Could you check a few things on this model? Use its own coordinates, in mm. Round coordinates to 2 decimals unless told otherwise and drop trailing zeros. Order: outer loops, then holes, each group sorted by start corner. A loop starts at its lowest first (then second) coordinate and runs counter-clockwise, first axis right, second up. Notation, with made-up numbers: (-23.75, -40) -> (-11.75, -40) arc R9 cw to (-11.75, -25) -> close; hole circle Ø6 at (-1, -37.75). An arc over 180 degrees is marked (long way). One line per question, with ' | ' between items.
```python
from build123d import *

# Parameters (mm, degrees)
SKETCH1_W                       = 38.1
SKETCH1_H                       = 19.05
EXTRUDE1_DEPTH                  = 142.875
M8X1_25_TAPPED_HOLE1_AT_2_COUNT = 2
M8X1_25_TAPPED_HOLE1_AT_2_PITCH = 25.4
M10X1_5_TAPPED_HOLE1_D          = 8.5
M5X0_8_TAPPED_HOLE2_D           = 4.2
M5X0_8_TAPPED_HOLE2_DEPTH       = 12.3952
M5X0_8_TAPPED_HOLE2_TIP         = 1.2618073
M5X0_8_TAPPED_HOLE3_D           = 4.2
M5X0_8_TAPPED_HOLE3_DEPTH       = 12.3952
M5X0_8_TAPPED_HOLE3_TIP         = 1.2618073


with BuildPart() as part:
    # Sketch1 → Extrude1 (new, symmetric)
    with BuildSketch(Plane(origin=(0, 0, 0), x_dir=(0, 0, -1), z_dir=(1, 0, 0))):
        Rectangle(SKETCH1_W, SKETCH1_H)
    extrude(amount=EXTRUDE1_DEPTH, both=True)

    # Sketch2 → M8x1.25 Tapped Hole1 (revolve, cut)
    with BuildSketch(Plane(origin=(142.875, 0, 12.7), x_dir=(0, 0, -1), z_dir=(0, 1, 0))):
        Polygon((0, 0), (0, 21.804126105), (3.4, 19.7612), (3.4, 0), align=None)
    m8x1_25_tapped_hole1 = revolve(axis=Axis((149.225, 0, 12.7), (-1, 0, 0)), mode=Mode.SUBTRACT)

    # M8x1.25 Tapped Hole1 at 2: M8x1.25 Tapped Hole1 ×2
    with Locations(*[(0, 0, -i * M8X1_25_TAPPED_HOLE1_AT_2_PITCH) for i in range(1, M8X1_25_TAPPED_HOLE1_AT_2_COUNT)]):
        add(m8x1_25_tapped_hole1, mode=Mode.SUBTRACT)

    # Mirror1: M8x1.25 Tapped Hole1 across plane
    add(m8x1_25_tapped_hole1.mirror(Plane(origin=(0, 0, 0), x_dir=(0, 0, 1), z_dir=(1, 0, 0))), mode=Mode.SUBTRACT)

    # Mirror1 copy 1 sketch → Mirror1 copy 1 (revolve, cut)
    with BuildSketch(Plane(origin=(-142.875, 0, -12.7), x_dir=(0, 0, -1), z_dir=(0, 1, 0))):
        Polygon((0, 0), (0, -21.804126105), (3.4, -19.7612), (3.4, 0), align=None)
    revolve(axis=Axis((-149.225, 0, -12.7), (-1, 0, 0)), mode=Mode.SUBTRACT)

    # M10x1.5 Tapped Hole1 (through all)
    with Locations(Plane(origin=(0, 9.525, 0), x_dir=(-1, 0, 0), z_dir=(0, 1, 0))):
        with Locations((47.625, 0), (-47.625, 0)):
            Hole(M10X1_5_TAPPED_HOLE1_D / 2)

    # M5x0.8 Tapped Hole2
    with Locations(Plane(origin=(-9.051259955, 7.173736758, -19.05), x_dir=(1, 0, 0), z_dir=(0, 0, -1))):
        with Locations((72.551259955, 7.173736758), (-54.448740045, 7.173736758)):
            Hole(M5X0_8_TAPPED_HOLE2_D / 2, depth=M5X0_8_TAPPED_HOLE2_DEPTH)
            with Locations((0, 0, -(M5X0_8_TAPPED_HOLE2_DEPTH + M5X0_8_TAPPED_HOLE2_TIP / 2))):  # 118° drill point
                Cone(0, M5X0_8_TAPPED_HOLE2_D / 2, M5X0_8_TAPPED_HOLE2_TIP, mode=Mode.SUBTRACT)

    # M5x0.8 Tapped Hole3
    with Locations(Plane(origin=(0, -9.525, 0), x_dir=(-1, 0, 0), z_dir=(0, -1, 0))):
        with Locations((-19.05, 12.7), (19.05, 12.7), (19.05, -12.7), (-19.05, -12.7)):
            Hole(M5X0_8_TAPPED_HOLE3_D / 2, depth=M5X0_8_TAPPED_HOLE3_DEPTH)
            with Locations((0, 0, -(M5X0_8_TAPPED_HOLE3_DEPTH + M5X0_8_TAPPED_HOLE3_TIP / 2))):  # 118° drill point
                Cone(0, M5X0_8_TAPPED_HOLE3_D / 2, M5X0_8_TAPPED_HOLE3_TIP, mode=Mode.SUBTRACT)


solid = part.part
```
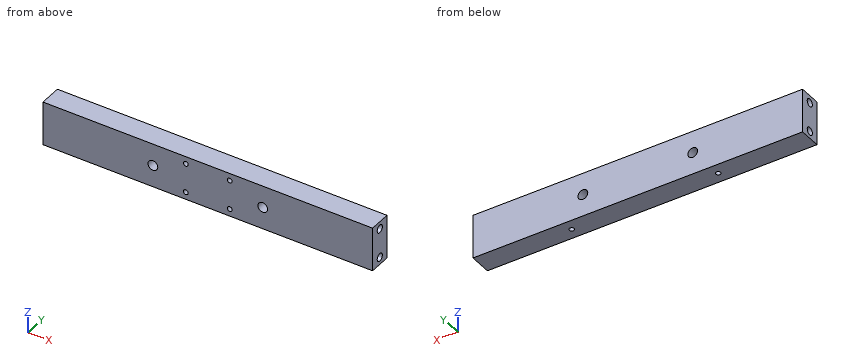
1. I need wall thicknesses on probe 1 along X at (y, z) = (0.25, -7) (3 decimals); probe 2 along Y at (x, z) = (133, -12.7) (3 decimals); probe 3 along Y at (x, z) = (-63, -12) (3 decimals). Which ranges of each line are inside material? Lowest first, please.
From the geometry:
probe 1: x = -142.875 to -65.585, -61.415 to 61.415, 65.585 to 142.875 | probe 2: y = -9.525 to -3.4, 3.4 to 9.525 | probe 3: y = -9.525 to -2.04, 2.04 to 9.525
2. I want a section at A-A on y = -5.75. List the corners of the cut face in (x, z) for me (3 decimals).
From the geometry:
outline: (-142.875, -19.05) -> (142.875, -19.05) -> (142.875, 19.05) -> (-142.875, 19.05) -> close; hole circle Ø8.5 at (-47.625, 0); hole circle Ø4.2 at (-19.05, -12.7); hole circle Ø4.2 at (-19.05, 12.7); hole circle Ø4.2 at (19.05, -12.7); hole circle Ø4.2 at (19.05, 12.7); hole circle Ø8.5 at (47.625, 0)
3. I'm going to push flat-ended pins straight in: pin 1 (6 mm diameter, centred on y = 0, z = 12.7, fed in from +X); pin 2 (7.5 mm diameter, centred on x = 47.625, z = 0, fed in from -Y); pin 3 (2.5 mm diameter, centred on x = 19.05, z = -12.7, fed in from -Y). Where does each tip first touch, or does it pass through?
From the geometry:
pin 1: stops at x = 122.87 | pin 2: passes through | pin 3: stops at y = 3.38
